Could you check a few things on this model? Use its own coordinates, in mm. Coordinates: 2 decimals unless noted, no trailing zeros. Loops run counter-clockwise (first coordinate to the right, second up) from the corner with the lowest first, then second, coordinate; pieces in that order, holes last. Notation, with made-up numbers: M -6.75,-10 L 10.25,-10 A3 ccw 10.25,-6 Z; hole C -11,-23.5 d8. An arc over 180 degrees is marked long. Use one line per item in the form item = value. Start each with the question number.
```python
from build123d import *

# Parameters (mm, degrees)
F0_R     = 46.181054
F0_R_2   = 26.367937
F1_DEPTH = 50.8
F2_SIZE  = 5.08
F3_R     = 5.08


with BuildPart() as f1:
    # F0 (on Top) → F1 (new body)
    with BuildSketch(Plane.XY):
        Circle(F0_R)
        Circle(F0_R_2, mode=Mode.SUBTRACT)
    extrude(amount=F1_DEPTH)

    # F2
    f2_edges = [f1.edges().sort_by_distance(p)[0] for p in [
        (-46.181054, 0, 50.8),
    ]]
    chamfer(f2_edges, length=F2_SIZE)

    # F3
    f3_edges = [f1.edges().sort_by_distance(p)[0] for p in [
        (-46.181054, 0, 0),
    ]]
    fillet(f3_edges, radius=F3_R)


solid = f1.part
```
Item 1: Please list where these lines run through material, in increasing order: line 1 along Y through (x, z) = (0, 36.5); line 2 along X through (y, z) = (-0.5, 19); line 3 along Y through (x, z) = (5, 30.5).
Item 2: Thinking about a two-plate mould opening in Y: for faces 1 (the flat face through (-1, -27, 50.8)), 2 (the conical face through (-8.963, -40.364, 50.553)), 3 (the cylindrical face through (25.15, 7.92, 25.04)), which applies, pulls with the +Y half, pulls with the -Y half, needs draft (parallel to the pull), parting line crosses it, or undercut?
Item 3: I'm going to push flat-ended pins straight in: P1, Ø8, axis at x = -33, z = 26.5, coming from the +Y side; P2, Ø12, axis at y = -27, z = 41.5, coming from the +X side; P3, Ø1.5, axis at y = 16.5, z = 6.5, coming from the -X side. Where does each tip first touch, or does it pass through?
Item 4: I want a section at C-C (z = 39.5). Write out the boundary of the cut face in (x, y).
Item 5: I want a section at A-A (y = 0). Write out the boundary of the cut face in (x, z), plus the area to 3 significant figures.
Worked answers:
q1.line_1 = -46.18 to -26.37, 26.37 to 46.18
q1.line_2 = -46.18 to -26.36, 26.36 to 46.18
q1.line_3 = -45.91 to -25.89, 25.89 to 45.91
q2.face_1 = needs draft
q2.face_2 = parting line crosses it
q2.face_3 = undercut
q3.P1 = 35.94
q3.P2 = 41.13
q3.P3 = -43.41
q4.outline = C 0,0 d92.36; hole C 0,0 d52.74
q5.outline = M -46.18,5.08 A5.08 ccw -41.1,0 L -26.37,0 L -26.37,50.8 L -41.1,50.8 L -46.18,45.72 Z; M 26.37,0 L 41.1,0 A5.08 ccw 46.18,5.08 L 46.18,45.72 L 41.1,50.8 L 26.37,50.8 Z
q5.area = 1,980 mm²
